from build123d import *

# Parameters (mm, degrees)
SKETCH003_R       = 1.375
EXTRUDE004_DEPTH  = 10
SKETCH001_R       = 0.9
EXTRUDE_DEPTH     = 2
SKETCH_R          = 3.9
EXTRUDE001_DEPTH  = 2
CYLINDER001_R     = 45
CYLINDER001_DEPTH = 7
CYLINDER_R        = 50
CYLINDER_DEPTH    = 9


with BuildPart() as extrude004:
    # Sketch003 (on Face6 of Extrude002) → Extrude004 (new body)
    with BuildSketch(Plane.XY.offset(14)):
        with Locations((-12.541029, 32.340019)):
            Circle(SKETCH003_R)
        with Locations((-5.469961, 39.411087)):
            Circle(SKETCH003_R)
        with Locations((5.225029, 21.645029)):
            Circle(SKETCH003_R)
    extrude(amount=-EXTRUDE004_DEPTH)


with BuildPart() as screwholes_middle_outer:
    # Sketch001 (on Face3 of Cut001) → Extrude (new body)
    with BuildSketch(Plane.XY.offset(9)):
        with Locations((0, 7.15)):
            Circle(SKETCH001_R)
        with Locations((-7.15, 0)):
            Circle(SKETCH001_R)
        with Locations((0, -7.15)):
            Circle(SKETCH001_R)
        with Locations((7.15, 0)):
            Circle(SKETCH001_R)
    extrude(amount=-EXTRUDE_DEPTH)


with BuildPart() as screwholes_middle_inner:
    # Sketch (on Face3 of Cut) → Extrude001 (new body)
    with BuildSketch(Plane.XY.offset(9)):
        Circle(SKETCH_R)
    extrude(amount=-EXTRUDE001_DEPTH)


with BuildPart() as cylinder001:
    # Cylinder001 → Cylinder001 (new body)
    with BuildSketch(Plane.XY):
        Circle(CYLINDER001_R)
    extrude(amount=CYLINDER001_DEPTH)


with BuildPart() as platform_shoulder_screws:
    # Cylinder → Cylinder (new body)
    with BuildSketch(Plane.XY):
        Circle(CYLINDER_R)
    extrude(amount=CYLINDER_DEPTH)

    # Cut: cut Cylinder001
    add(cylinder001.part, mode=Mode.SUBTRACT)

    # Cut001: cut Screwholes-middle-inner
    add(screwholes_middle_inner.part, mode=Mode.SUBTRACT)

    # Cut002: cut Screwholes-middle-outer
    add(screwholes_middle_outer.part, mode=Mode.SUBTRACT)

    # Cut003: cut Extrude004
    add(extrude004.part, mode=Mode.SUBTRACT)


solid = platform_shoulder_screws.part
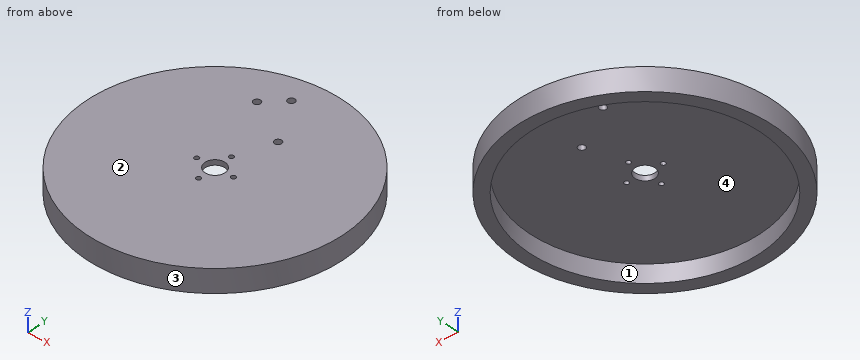
Geometry check sheet. Reference: the model listing, model coordinates, mm. Face numbers are marked on the shaded views. Round coordinates to 2 decimals unless told otherwise and drop trailing zeros. Order: outer loops, then holes, each group sorted by start corner. A loop starts at its lowest first (then second) coordinate and runs counter-clockwise, first axis right, second up. Notation, with made-up numbers: M 31.25,-2.5 L 44.25,-2.5 A17 ccw 44.25,8.5 Z; hole C 31.5,68.25 d7. An arc over 180 degrees is marked long. Write each question's results on one line, items separated by ' | '. Start each with the question number.
1. Cross-section at C-C on z = 1.5. Record the boundary of the cut face in (x, y), plus the area to 3 significant figures.
2. Draft check along Y on the marked faces 1, 2, 3 and 4. Enter one of: pulls with the +Y half, pulls with the -Y half, needs draft (parallel to the pull), parting line crosses it, or undercut.
3. Cross-section at A-A on y = 2.5. Record the boundary of the cut face in (x, z), plus the area to 3 significant figures.
4. Cross-section at D-D on y = -31. Record the boundary of the cut face in (x, z).
5. Cross-section at B-B on x = -26.5. Record the boundary of the cut face in (y, z), plus the area to 3 significant figures.
6. Go/stop test with flat-tipped pins: P1, Ø3, axis at x = -8.5, z = 2, coming from the -Y side; P2, Ø5, axis at y = 16, z = 8, coming from the +X side; P3, Ø3, axis at x = 0, y = 7.15, coming from the -Z side. Record where each tip stops, or that it passes through.
7. Material ranges on L1, parallel to Y at x = 0, z = 8.45; L2, parallel to Z at x = -1, y = -34.5; L3, parallel to X at y = 22.5, z = 1, recorded low to high. Write a range as from..to.
Resolved:
1) outline: C 0,0 d100; hole C 0,0 d90 | area: 1,490 mm2
2) face 1: undercut | face 2: needs draft | face 3: parting line crosses it | face 4: undercut
3) outline: M -49.94,0 L -44.93,0 L -44.93,7 L -2.99,7 L -2.99,9 L -49.94,9 Z; M 2.99,7 L 44.93,7 L 44.93,0 L 49.94,0 L 49.94,9 L 2.99,9 Z | area: 258 mm2
4) outline: M -39.23,0 L -32.62,0 L -32.62,7 L 32.62,7 L 32.62,0 L 39.23,0 L 39.23,9 L -39.23,9 Z
5) outline: M -42.4,0 L -36.37,0 L -36.37,7 L 36.37,7 L 36.37,0 L 42.4,0 L 42.4,9 L -42.4,9 Z | area: 254 mm2
6) P1: y = -49.51 | P2: x = 48.14 | P3: z = 7
7) L1: -50..-8.05, -6.25..-3.9, 3.9..6.25, 8.05..50 | L2: 7..9 | L3: -44.65..-38.97, 38.97..44.65
